from build123d import *

# Parameters (mm, degrees)
F0_W     = 152.4
F0_H     = 127
F1_DEPTH = 63.5
F2_W     = 101.6
F2_H     = 76.2
F3_DEPTH = 76.2
F4_R     = 50.8
F5_R     = 30.648749
F6_DEPTH = 38.1
F7_W     = 50.8
F7_H     = 50.8
F8_DEPTH = 50.8
F9_SIZE  = 25.4


with BuildPart() as f1:
    # F0 (on Top) → F1 (new body, symmetric)
    with BuildSketch(Plane.XY):
        Rectangle(F0_W, F0_H)
    extrude(amount=F1_DEPTH, both=True)

    # F2 (on face) → F3 (cut)
    with BuildSketch(Plane.XY.offset(63.5)):
        with Locations((25.4, -25.4)):
            Rectangle(F2_W, F2_H)
    extrude(amount=-F3_DEPTH, mode=Mode.SUBTRACT)

    # F4
    f4_edges = [f1.edges().sort_by_distance(p)[0] for p in [
        (-50.8, -63.5, 63.5),
    ]]
    fillet(f4_edges, radius=F4_R)

    # F5 (on face) → F6 (cut)
    with BuildSketch(Plane.XY.offset(-12.7)):
        with Locations((28.892498, -27.33675)):
            Circle(F5_R)
    extrude(amount=-F6_DEPTH, mode=Mode.SUBTRACT)

    # F7 (on face) → F8 (cut)
    with BuildSketch(Plane.XY.offset(63.5)):
        with Locations((0, 38.1)):
            Rectangle(F7_W, F7_H)
    extrude(amount=-F8_DEPTH, mode=Mode.SUBTRACT)

    # F9
    f9_edges = [f1.edges().sort_by_distance(p)[0] for p in [
        (76.2, 38.1, 63.5),
    ]]
    chamfer(f9_edges, length=F9_SIZE)


solid = f1.part
For this review, take the finished solid that the model builds, in its own axes (mm). A direction names the side the tool comes from. Give positions to 0.01 mm unless a question says otherwise; leave off trailing zeros. Write each loop counter-clockwise with the first axis right and the second up, starting at its lowest first coordinate (ties: lowest second). Pieces come first, ordered by that corner, then holes. Notation, with made-up numbers: (35.5, 59.25) -> (46.5, 59.25) arc R20 ccw to (46.5, 66.25) -> close; hole circle Ø11 at (-39.5, 10.5). An arc over 180 degrees is marked (long way). Use CSV: the item, a comma, the result in double quotes.
Q1. Mouldability with a two-part tool opening along Y and no side actions: class faces 5 (the face through (36, 12.7, 17)), 6 (the face through (-1, 63.5, 1)), 7 (the face through (25.4, 38, 38)), 8 (the face through (6.303, -6.623, -31.483)) as pulls with the +Y half, pulls with the -Y half, needs draft (parallel to the pull), parting line crosses it, or undercut.
Conclusion:
face 5,"pulls with the -Y half"
face 6,"pulls with the +Y half"
face 7,"needs draft"
face 8,"undercut"
Q2. Take a section at B-B, the plane x = -32. Write out the cut boundary in (y, z).
Conclusion:
outline,"(-63.5, -63.5) -> (63.5, -63.5) -> (63.5, 63.5) -> (-12.7, 63.5) arc R50.8 ccw to (-63.5, 12.7) -> close"
Q3. Take a section at A-A, the plane z = 22. Write out the cut boundary in (x, y), then the cut area to 3 significant figures.
Conclusion:
outline,"(-76.2, -62.64) -> (-25.4, -62.64) -> (-25.4, 63.5) -> (-76.2, 63.5) -> close; (25.4, 12.7) -> (76.2, 12.7) -> (76.2, 63.5) -> (25.4, 63.5) -> close"
area,"8,990 mm2"
Q4. For P1, Ø1, axis at x = -28.5, y = -17.5, coming from the +Z side; P2, Ø10, axis at x = 57.5, y = -32.5, coming from the +Z side; P3, Ø2, axis at x = -39.5, z = 18.5, coming from the -Y side, all flat-tipped, find the tip position at first contact; note any pin that passes through.
Conclusion:
P1,"z = 63.32"
P2,"z = -12.7"
P3,"y = -63.27"
Q5. Tool access review of faces 1 (the face through (0, 38, 12.7)), 2 (the face through (28, -27, -50.8)), 3 (the face through (2, -8, -12.7)), 4 (the face through (-25.4, -1, 26)): name each direction out of +Z, -Z, +X, -X, +Y, -Y from which nothing blocks a thin tool from reaching the whole face with its end or side.
Conclusion:
face 1,"+Z, +Y, -Y"
face 2,"+Z"
face 3,"+Z, +X, -Y"
face 4,"+Z, -Y"
Q6. To check wall thickness, follow probe 1 along X at (y, z) = (28, 22.5); probe 2 along Y at (x, z) = (50, 30.5); probe 3 along Z at (x, y) = (3.5, -40). State the ranges of each line that lie inside material, in increasing order. Write a range as [from, to].
Conclusion:
probe 1,"[-76.2, -25.4], [25.4, 76.2]"
probe 2,"[12.7, 63.5]"
probe 3,"[-63.5, -50.8]"
Q7. Take a section at C-C, the plane z = -2. Write out the cut boundary in (x, y), then the cut area to 3 significant figures.
Conclusion:
outline,"(-76.2, -63.5) -> (-25.4, -63.5) -> (-25.4, 12.7) -> (76.2, 12.7) -> (76.2, 63.5) -> (-76.2, 63.5) -> close"
area,"11,600 mm2"
Q8. Take a section at D-D, the plane y = 37. Write out the cut boundary in (x, z), then the cut area to 3 significant figures.
Conclusion:
outline,"(-76.2, -63.5) -> (76.2, -63.5) -> (76.2, 38.1) -> (50.8, 63.5) -> (25.4, 63.5) -> (25.4, 12.7) -> (-25.4, 12.7) -> (-25.4, 63.5) -> (-76.2, 63.5) -> close"
area,"16,500 mm2"
